Geometry check sheet. Reference: the model listing, model coordinates, mm. A direction names the side the tool comes from. Coordinates: 2 decimals unless noted, no trailing zeros. Write each loop counter-clockwise with the first axis right and the second up, starting at its lowest first coordinate (ties: lowest second). Pieces come first, ordered by that corner, then holes. Notation, with made-up numbers: (43.25, 43) -> (74.25, 43) arc R25 ccw to (74.25, 66) -> close; hole circle Ø11 at (56.25, -35). An arc over 180 degrees is marked (long way). Put each result on its own line as item: value. Start each with the question number.
Autodesk Inventor part; units mm, degrees
ref_plane "YZ Plane" through (0, 0, 0) normal (1, 0, 0) x (0, 1, 0)
ref_plane "XZ Plane" through (0, 0, 0) normal (0, 1, 0) x (-1, 0, 0)
ref_plane "XY Plane" through (0, 0, 0) normal (0, 0, 1) x (1, 0, 0)
sketch "Sketch1" plane through (0, 0, 0) normal (0, 1, 0) x (-1, 0, 0)
  line L0 (18.2162, 26.4548) -> (-7.1838, 26.4548)
  line L1 (-7.1838, 26.4548) -> (-7.1838, -24.3452)
  line L2 (-7.1838, -24.3452) -> (18.2162, -24.3452)
  line L3 (18.2162, -24.3452) -> (18.2162, 26.4548)
  point P0 (0, 0)
  dimension "d0" = 50.8
  dimension "d1" = 25.4
extrude "Extrusion1" add sketch "Sketch1" along normal blind 2.54
sketch "Sketch2" plane through (7.1838, 0, -24.3452) normal (0, 0, -1) x (-1, 0, 0)
  line L0 (0, 0) -> (73.3235, -127)
  line L1 (73.3235, -127) -> (98.7235, -127)
  line L2 (0, 0) -> (25.4, 0)
  line L3 (98.7235, -127) -> (25.4, 0)
  line L4 (0, 2.54) -> (25.4, 2.54)
  line L5 (0, 0) -> (0, 2.54)
  line L6 (0, 2.54) -> (25.4, 2.54)
  line L7 (25.4, 2.54) -> (25.4, 0)
  point P0 (7.1838, 0)
  dimension "d4" = 60
  dimension "d5" = 127
extrude "Extrusion2" add sketch "Sketch2" along normal blind 2.54
sketch "Sketch3" plane through (-18.2162, 0, 26.4548) normal (0, 0, 1) x (1, 0, 0)
  line L0 (0, 0) -> (0, 2.54)
  line L1 (0, 0) -> (0, 2.54)
  line L2 (25.4, 0) -> (25.4, 2.54)
  line L3 (0, 2.54) -> (25.4, 2.54)
  line L4 (25.4, 2.54) -> (25.4, 0)
  line L5 (25.4, 0) -> (-47.9235, -127)
  line L6 (25.4, 0) -> (-47.9235, -127)
  line L7 (-47.9235, -127) -> (-73.3235, -127)
  line L8 (-47.9235, -127) -> (-73.3235, -127)
  line L9 (-73.3235, -127) -> (0, 0)
  point P0 (18.2162, 0)
extrude "Extrusion3" add sketch "Sketch3" along normal blind 2.54
sketch "Sketch4" plane through (0, 2.54, 0) normal (0, 1, 0) x (1, 0, 0)
  line L0 (7.1838, -26.4548) -> (7.1838, 24.3452) construction
  line L1 (-66.1396, -28.9948) -> (7.1838, -28.9948) construction
  line L2 (7.1838, -1.0548) -> (-9.3262, -1.0548) construction
  line L3 (-9.3262, -1.0548) -> (-9.3262, -28.9948) construction
  line L4 (-9.3262, -28.9948) -> (7.1838, -28.9948) construction
  line L5 (7.1838, -28.9948) -> (7.1838, -1.0548) construction
  circle A0 centre (-9.3262, -1.0548) radius 4.7625
  dimension "d11" = 16.51
  dimension "d12" = 9.525
extrude "Extrusion4" add sketch "Sketch4" along normal blind 76.2
sketch "Sketch5" plane through (7.1838, 0, -26.8852) normal (0, 0, -1) x (-1, 0, 0)
  line L0 (98.7235, -127) -> (25.4, 0)
  line L1 (98.7235, -127) -> (75.8635, -127)
  line L2 (75.8635, -127) -> (75.8635, -87.4053)
  line L3 (75.8635, -87.4053) -> (98.7235, -87.4053)
  line L4 (98.7235, -87.4053) -> (98.7235, -127)
  circle A0 centre (75.8635, -122.2375) radius 3.175
  circle A1 centre (75.8635, -113.9825) radius 3.175
  circle A2 centre (75.8635, -105.7275) radius 3.175
  circle A3 centre (75.8635, -97.4725) radius 3.175
  point P0 (7.1838, 0)
  dimension "d15" = 6.35
  dimension "d16" = 4.7625
  dimension "d17" = 22.86
  dimension "d20" = 8.255
extrude "Extrusion5" cut sketch "Sketch5" against normal through all contours A3 L2 | L2 A3 | A0 L2 | L2 A0 | A2 L2 | L2 A2 | A1 L2 | L2 A1
sketch "Sketch6" plane through (-18.2162, 0, 28.9948) normal (0, 0, 1) x (1, 0, 0)
  circle A0 centre (-50.4635, -105.7275) radius 3.175
  circle A1 centre (-50.4635, -105.7275) radius 101.6 construction
  line L0 (25.4, 2.54) -> (0, 2.54)
  point P0 (18.2162, 0)
  point P1 (-50.4635, -4.1275)
  dimension "d27" = 203.2
  dimension "d28" = 6.6675
properties part number "Wheel-Housing"
Item 1: Section check A-A, the plane y = -14. Enter the section's corners in (x, z).
Item 2: Mould release check, pull along Y, two halves, no side actions. Record for faces 4 (the flat face through (-55.39, -64.39, -25.6)), 5 (the flat face through (-28.965, -62.611, -25.597)), 6 (the cylindrical face through (-68.266, -110.835, 27.707)): released by +Y, released by -Y, zero draft, split by the parting line, or undercut.
Item 3: Scan lines: line 1 along Z through (x, y) = (-45, -64); line 2 along Y through (x, z) = (-8.5, 7); line 3 along Z through (x, y) = (-10, 33.5). Record each from-to range of solid material in increasing order. Write a range as [from, to].
Item 4: Section check D-D, the plane y = 59.5. Enter the section's corners in (x, z) (1 decimal), and give its area (3 significant figures).
Item 5: Access from +Z, -Z, +X, -X, +Y, -Y to the whole of each face (thin tool, end or side, straight path). Record for faces 1 (the flat face through (-42, -58, -24.345)), 2 (the cylindrical face through (-4.784, 40.107, 2.485)), 3 (the cylindrical face through (-70.387, -94.795, 27.707)).
Item 6: Section check B-B, the plane x = -27.5. Enter the section's corners in (y, z), and give its area (3 significant figures).
Item 7: Section check C-C, the plane z = -8.5. Enter the section's corners in (x, y), and give its area (3 significant figures).
Item 8: Go/stop test with flat-tipped pins: P1, Ø5, axis at x = -68.68, y = -97.47, coming from the +Z side; P2, Ø0.8, axis at y = 1, z = -8, coming from the -X side; P3, Ø12.5, axis at x = -11.5, z = 7, coming from the -Y side. Record where each tip stops, or that it passes through.
From the geometry:
1. outline: (-26.3, -26.89) -> (-0.9, -26.89) -> (-0.9, -24.35) -> (-26.3, -24.35) -> close; (-26.3, 26.45) -> (-0.9, 26.45) -> (-0.9, 28.99) -> (-26.3, 28.99) -> close
2. face 4: released by +Y
2. face 5: released by -Y
2. face 6: undercut
3. line 1: [-26.89, -24.35], [26.45, 28.99]
3. line 2: [0, 2.54]
3. line 3: [-3.66, 5.77]
4. outline: circle Ø9.5 at (-9.3, 1.1)
4. area: 71.3 mm²
5. face 1: +X, -X, -Y
5. face 2: +Y
5. face 3: +Z, -Z
6. outline: (-60.07, -26.89) -> (-16.08, -26.89) -> (-16.08, -24.35) -> (-60.07, -24.35) -> close; (-60.07, 26.45) -> (-16.08, 26.45) -> (-16.08, 28.99) -> (-60.07, 28.99) -> close
6. area: 223 mm²
7. outline: (-18.22, 0) -> (7.18, 0) -> (7.18, 2.54) -> (-18.22, 2.54) -> close
7. area: 64.5 mm²
8. P1: through
8. P2: x = -18.22
8. P3: y = 0
